Can you work these out from the model? Positions are in its coordinate system, mm. Face numbers are marked on the shaded views. Coordinates: 2 decimals unless noted, no trailing zeros. Write each loop counter-clockwise with the first axis right and the second up, starting at its lowest first coordinate (ties: lowest second). Pieces come first, ordered by that corner, then holes. Notation, with made-up numbers: M 27,11 L 66,11 A28 cw 66,31 Z; hole C 0.25,47 d11. An arc over 180 degrees is marked long. Use one line per item in the form item = value. Start each with the question number.
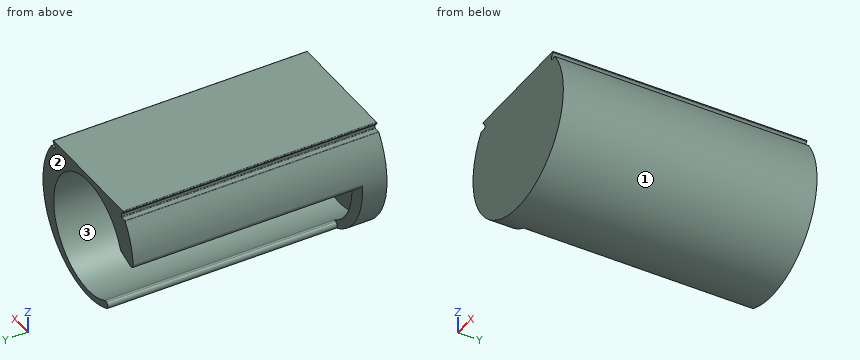
```python
from build123d import *

# Parameters (mm, degrees)
SKETCH1_R           = 16.4
BOSS_EXTRUDE1_DEPTH = 70
BOSS_EXTRUDE2_START = 0.8
BOSS_EXTRUDE2_DEPTH = 0.8
CUT_EXTRUDE1_DEPTH  = 64
FILLET1_R           = 1
FILLET2_R           = 0.2


with BuildPart() as part:
    # Sketch1 → Boss-Extrude1 (new body)
    with BuildSketch(Plane(origin=(0, 0, 0), x_dir=(1, 0, 0), z_dir=(0, 1, 0))):
        with BuildLine():
            Line((-18.386301809, -27.686071188), (-20.098433843, -27.686071188))
            Line((-20.098433843, -27.686071188), (-20.098433843, -28.698203222))
            Line((-20.098433843, -28.698203222), (-19.298433843, -29.498203222))
            Line((-19.298433843, -29.498203222), (-19.298433843, -29.886071188))
            Line((-19.298433843, -29.886071188), (-52.598433843, -29.886071188))
            Line((-52.598433843, -29.886071188), (-52.598433843, -29.498203222))
            Line((-52.598433843, -29.498203222), (-51.798433843, -28.698203222))
            Line((-51.798433843, -28.698203222), (-51.798433843, -27.686071188))
            Line((-51.798433843, -27.686071188), (-53.510565878, -27.686071188))
            ThreePointArc((-53.510565878, -27.686071188), (-35.948433843, 6.216409145), (-18.386301809, -27.686071188))
        make_face()
        with Locations(Location((-35.948433843, -11.886071188, 0), (0, 0, 270))):
            Circle(SKETCH1_R, mode=Mode.SUBTRACT)
    extrude(amount=BOSS_EXTRUDE1_DEPTH)

    # Sketch2 → Boss-Extrude2 (add)
    with BuildSketch(Plane.XZ.offset(BOSS_EXTRUDE2_START)):
        with BuildLine():
            Line((-18.386301809, 27.686071188), (-20.098433843, 27.686071188))
            Line((-20.098433843, 27.686071188), (-20.098433843, 28.698203222))
            Line((-20.098433843, 28.698203222), (-19.298433843, 29.498203222))
            Line((-19.298433843, 29.498203222), (-19.298433843, 29.886071188))
            Line((-19.298433843, 29.886071188), (-52.598433843, 29.886071188))
            Line((-52.598433843, 29.886071188), (-52.598433843, 29.498203222))
            Line((-52.598433843, 29.498203222), (-51.798433843, 28.698203222))
            Line((-51.798433843, 28.698203222), (-51.798433843, 27.686071188))
            Line((-51.798433843, 27.686071188), (-53.510565878, 27.686071188))
            ThreePointArc((-53.510565878, 27.686071188), (-35.948433843, -6.216409145), (-18.386301809, 27.686071188))
        make_face()
    extrude(amount=-BOSS_EXTRUDE2_DEPTH)

    # Sketch3 → Cut-Extrude1 (cut)
    with BuildSketch(Plane(origin=(0, 70, 0), x_dir=(1, 0, 0), z_dir=(0, 1, 0))):
        Polygon((-49.615972348, -18.085360607), (-42.433549338, 1.648184429), (-57.414050135, 7.100640814), (-64.596473145, -12.632904223), align=None)
    extrude(amount=-CUT_EXTRUDE1_DEPTH, mode=Mode.SUBTRACT)

    # Fillet1
    fillet1_edges = [part.edges().sort_by_distance(p)[0] for p in [
        (-44.195484744, 38, -2.289476472),
        (-51.377907754, 38, 17.444068565),
        (-57.448378022, 38, 15.234598079),
        (-46.841576343, 38, -3.252575051),
    ]]
    fillet(fillet1_edges, radius=FILLET1_R)

    # Fillet2
    fillet2_edges = [part.edges().sort_by_distance(p)[0] for p in [
        (-18.386301809, 34.6, 27.686071188),
        (-20.098433843, 34.6, 27.686071188),
        (-20.098433843, 34.6, 28.698203222),
        (-19.298433843, 34.6, 29.498203222),
        (-19.298433843, 34.6, 29.886071188),
        (-52.598433843, 34.6, 29.886071188),
        (-52.598433843, 34.6, 29.498203222),
        (-51.798433843, 34.6, 28.698203222),
        (-51.798433843, 34.6, 27.686071188),
        (-53.510565878, 34.6, 27.686071188),
    ]]
    fillet(fillet2_edges, radius=FILLET2_R)


solid = part.part
```
1) Suppose I cut it at C-C on x = -38.5. Please give me the cut outline in (y, z).
2) Suppose I cut it at B-B on y = 4.5. Please give me the cut outline in (x, z), and give its area (3 significant figures).
3) Suppose I cut it at A-A on z = 1.5. Please give me the cut outline in (x, y).
4) If we mould it in two halves opening along X, with no side actions, what happens to the marked faces 1, 2 and 3? For each: +X half, -X half, draft (parallel to the pull), parting line (faces both ways), or undercut.
5) Suppose I cut it at D-D on y = 20.5. Please give me the cut outline in (x, z), and give its area (3 significant figures).
6) Will these pins go through, and if not, where does the flat tip stop? pin 1 Ø11 at (x, z) = (-52.5, 1.5) entering from +Y; pin 2 Ø2 at (x, z) = (-27.5, 21) entering from +Y; pin 3 Ø10 at (y, z) = (44.5, 24.5) entering from +X.
7) Please list where these lines run through material, in increasing order: line 1 (Z direction, x = -35.5, y = 11); line 2 (Y direction, x = -46, z = 23); line 3 (X direction, y = 34, z = 22).
Computed values:
q1.outline = M -0.8,-6.06 L 70,-6.06 L 70,-4.31 L 0,-4.31 L 0,28.09 L 70,28.09 L 70,29.89 L -0.8,29.89 Z
q2.outline = M -53.57,27.6 A21.5 ccw long -18.33,27.6 A0.2 ccw -18.49,27.69 L -19.9,27.69 A0.2 cw -20.1,27.89 L -20.1,28.62 A0.2 cw -20.04,28.76 L -19.36,29.44 A0.2 ccw -19.3,29.58 L -19.3,29.69 A0.2 ccw -19.5,29.89 L -52.4,29.89 A0.2 ccw -52.6,29.69 L -52.6,29.58 A0.2 ccw -52.54,29.44 L -51.86,28.76 A0.2 cw -51.8,28.62 L -51.8,27.89 A0.2 cw -52,27.69 L -53.41,27.69 A0.2 ccw Z; hole C -35.95,11.89 d32.8
q2.area = 454 mm²
q3.outline = M -52.45,-0.8 L -19.45,-0.8 L -19.45,70 L -23.26,70 L -23.26,0 L -48.64,0 L -48.64,6 L -52.45,6 Z
q4.face_1 = parting line
q4.face_2 = draft
q4.face_3 = undercut
q5.outline = M -57.4,16.75 A1 ccw -56.06,15.74 L -51.81,17.29 A1 ccw -51.22,17.86 A16.4 cw long -43.81,-2.51 A1 ccw -44.63,-2.45 L -44.7,-2.47 A1 ccw -44.77,-4.32 A21.5 ccw -18.33,27.6 A0.2 ccw -18.49,27.69 L -19.9,27.69 A0.2 cw -20.1,27.89 L -20.1,28.62 A0.2 cw -20.04,28.76 L -19.36,29.44 A0.2 ccw -19.3,29.58 L -19.3,29.69 A0.2 ccw -19.5,29.89 L -52.4,29.89 A0.2 ccw -52.6,29.69 L -52.6,29.58 A0.2 ccw -52.54,29.44 L -51.86,28.76 A0.2 cw -51.8,28.62 L -51.8,27.89 A0.2 cw -52,27.69 L -53.41,27.69 A0.2 ccw -53.57,27.6 A21.5 ccw Z
q5.area = 369 mm²
q6.pin_1 = 6
q6.pin_2 = 0
q6.pin_3 = -14.87
q7.line_1 = -6.21 to -4.51, 28.28 to 29.89
q7.line_2 = -0.8 to 0
q7.line_3 = -56.37 to -48.86, -23.04 to -15.52
